Design review of the part built by this model. Coordinates are the model's own, in mm. A direction names the side the tool comes from. Coordinates: 2 decimals unless noted, no trailing zeros. Order: outer loops, then holes, each group sorted by start corner. A loop starts at its lowest first (then second) coordinate and runs counter-clockwise, first axis right, second up. Notation, with made-up numbers: (-22.75, -7) -> (2.25, -7) arc R26 ccw to (2.25, 8) -> close; hole circle Ø5 at (39, 6.25). An arc over 180 degrees is marked (long way). Use a Markdown table: item, result. Add a question column.
Q1. Add section A-A (y = 1.25). State the section outline as (x, z) points, then the cut area to 3 significant figures.
Q2. Add section B-B (y = 2.5). State the section outline as (x, z) points.
Q3. Insertion check: pin 1 (1 mm diameter, centred on x = 19.5, z = 1.5, fed in from -Y). The pin has a flat end and moves straight along its axis. Give the tip position at first contact, or say it passes through.
Q4. The part is to be moulded in two halves that separate along Z. For faces 1 (the face through (18, 2, 1)), 2 (the face through (19, 2.2, 1)), 3 (the face through (11, 6, 2.8)), say which applies: pulls with the +Z half, pulls with the -Z half, needs draft (parallel to the pull), parting line crosses it, or undercut.
Q5. Machinability: for faces 4 (the face through (21, 4, 1)), 5 (the face through (19, 1, 0.4)), 6 (the face through (3, 3, 1)), which of the approach directions +Z, -Z, +X, -X, +Y, -Y give a long, thin tool a straight path to every point of the face, cutting with its end or side? Answer none if there is none.
Q6. Wall thickness on probe 1 along X at (y, z) = (2, 0.45); probe 2 along X at (y, z) = (2, 0.2); probe 3 along Y at (x, z) = (12.5, 1.6): over which ranges is each line inside the solid? List them lowest first.
Q7. Add section C-C (x = 2). State the section outline as (y, z) points.
Q8. Add section D-D (z = 2). State the section outline as (x, y) points, then the cut area to 3 significant figures.
from build123d import *

# Parameters (mm, degrees)
BOSS_EXTRUDE1_DEPTH = 2.8
SKETCH2_W           = 2
SKETCH2_H           = 2
CUT_EXTRUDE1_DEPTH  = 2.2


with BuildPart() as part:
    # Sketch1 → Boss-Extrude1 (new body)
    with BuildSketch(Plane.XY):
        Polygon((0, 0), (0, 7), (21, 7), (21, 0), (18, 0), (18, 5), (3, 5), (3, 0), align=None)
    extrude(amount=BOSS_EXTRUDE1_DEPTH)

    # Sketch2 → Cut-Extrude1 (cut)
    with BuildSketch(Plane.XZ):
        with Locations((19.5, 1.4)):
            Rectangle(SKETCH2_W, SKETCH2_H)
        with Locations((1.5, 1.4)):
            Rectangle(SKETCH2_W, SKETCH2_H)
    extrude(amount=-CUT_EXTRUDE1_DEPTH, mode=Mode.SUBTRACT)


solid = part.part
Established:
| question | item | result |
|---|---|---|
| 1 | outline | (0, 0) -> (3, 0) -> (3, 2.8) -> (0, 2.8) -> close; (18, 0) -> (21, 0) -> (21, 2.8) -> (18, 2.8) -> close; hole (0.5, 0.4) -> (2.5, 0.4) -> (2.5, 2.4) -> (0.5, 2.4) -> close; hole (18.5, 0.4) -> (20.5, 0.4) -> (20.5, 2.4) -> (18.5, 2.4) -> close |
| 1 | area | 8.80 mm^2 |
| 2 | outline | (0, 0) -> (3, 0) -> (3, 2.8) -> (0, 2.8) -> close; (18, 0) -> (21, 0) -> (21, 2.8) -> (18, 2.8) -> close |
| 3 | pin 1 | y = 2.2 |
| 4 | face 1 | needs draft |
| 4 | face 2 | undercut |
| 4 | face 3 | pulls with the +Z half |
| 5 | face 4 | +Z, -Z, +X, +Y, -Y |
| 5 | face 5 | -Y |
| 5 | face 6 | +Z, -Z, -Y |
| 6 | probe 1 | 0 to 0.5, 2.5 to 3, 18 to 18.5, 20.5 to 21 |
| 6 | probe 2 | 0 to 3, 18 to 21 |
| 6 | probe 3 | 5 to 7 |
| 7 | outline | (0, 0) -> (7, 0) -> (7, 2.8) -> (0, 2.8) -> (0, 2.4) -> (2.2, 2.4) -> (2.2, 0.4) -> (0, 0.4) -> close |
| 8 | outline | (0, 0) -> (0.5, 0) -> (0.5, 2.2) -> (2.5, 2.2) -> (2.5, 0) -> (3, 0) -> (3, 5) -> (18, 5) -> (18, 0) -> (18.5, 0) -> (18.5, 2.2) -> (20.5, 2.2) -> (20.5, 0) -> (21, 0) -> (21, 7) -> (0, 7) -> close |
| 8 | area | 63.2 mm^2 |
